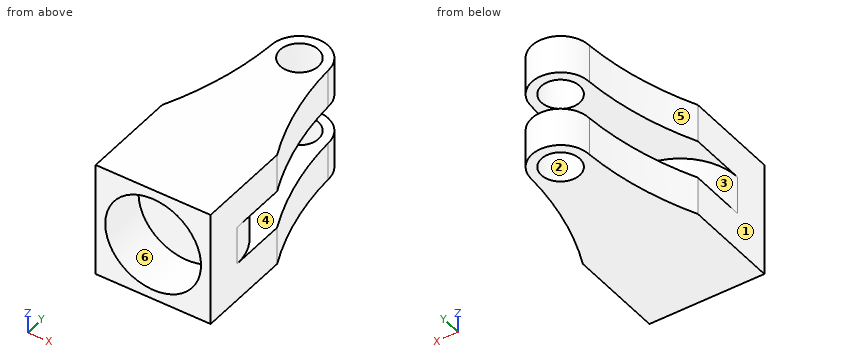
Autodesk Inventor part; units mm, degrees
ref_plane "Płaszczyzna konstrukcyjna2" through (-6, 5, 0) normal (0, 0, 1) x (1, 0, 0)
ref_plane "Płaszczyzna konstrukcyjna3" through (-6, -5, 0) normal (0, 0, 1) x (1, 0, 0)
ref_plane "YZ Plane" through (0, 0, 0) normal (1, 0, 0) x (0, 1, 0)
sketch "Szkic3" plane through (0, 0, 0) normal (0, 1, 0) x (-1, 0, 0)
  circle A0 centre (0, 0) radius 5
  line L0 (-6, -6) -> (6, -6)
  line L1 (6, -6) -> (6, 6)
  line L2 (6, 6) -> (-6, 6)
  line L3 (-6, 6) -> (-6, -6)
  line L4 (-6, -6) -> (6, 6) construction
  line L5 (6, -6) -> (-6, 6) construction
  dimension "d12" = 10
  dimension "d15" = 12
  dimension "d16" = 12
extrude "Wyciągnięcie proste3" add sketch "Szkic3" along normal mid plane 10
extrude "Wyciągnięcie proste4" add sketch "Szkic3" along normal blind 5 contours A0
ref_plane "Płaszczyzna konstrukcyjna2" through (-6, 5, 0) normal (0, 0, 1) x (1, 0, 0)
sketch "Szkic7" plane through (-6, 5, 0) normal (0, 0, 1) x (1, 0, 0)
  line L0 (0, -10) -> (0, 0)
  line L1 (0, 0) -> (12, 0)
  line L2 (12, 0) -> (6, 0)
  line L3 (6, 0) -> (6, 12) construction
  circle A0 centre (6, 12) radius 2
  line L4 (6, 12) -> (8, 12) construction
  line L5 (8, 12) -> (9, 12)
  line L6 (6, 12) -> (6, 14) construction
  line L7 (6, 14) -> (6, 15)
  arc A1 (9, 12) -> (6, 15) centre (6, 12) ccw
  arc A2 (9, 12) -> (12, 0) centre (41.9474, 13.8619) ccw
  line L8 (4, 12) -> (3, 12)
  arc A3 (6, 15) -> (3, 12) centre (6, 12) ccw
  arc A4 (0, 0) -> (3, 12) centre (-29.9474, 13.8619) ccw
  point P0 (6, -5)
  dimension "d61" = 12
  dimension "d62" = 4
  dimension "d63" = 1
  dimension "d64" = 2
  dimension "d65" = 1
  dimension "d66" = 3
  dimension "d67" = 33
  dimension "d68" = 1
  dimension "d69" = 2
  dimension "d70" = 3
  dimension "d71" = 33
extrude "Wyciągnięcie proste7" add sketch "Szkic7" along normal mid plane 12 contours A4 L8 A0 L5 A2 L1 | A3 L7 A0 L8 | A1 L5 A0 L7
ref_plane "Płaszczyzna konstrukcyjna3" through (-6, -5, 0) normal (0, 0, 1) x (1, 0, 0)
sketch "Szkic9" plane through (-6, -5, 0) normal (0, 0, 1) x (1, 0, 0)
  arc A0 (9, 22) -> (12, 10) centre (41.9474, 23.8619) ccw
  line L0 (0, 34) -> (12, 34)
  line L1 (12, 34) -> (12, 10)
  line L2 (12, 10) -> (0, 10)
  line L3 (0, 10) -> (0, 34)
  circle A1 centre (6, 22) radius 2
  line L4 (0, 34) -> (12, 10) construction
  line L5 (12, 34) -> (0, 10) construction
  point P0 (6, 5)
extrude "Wyciągnięcie proste9" cut sketch "Szkic9" along normal mid plane 4
fillet "Zaokrąglenie7" radius 6 2 edges at (6, 5, 0) (-6, 5, 0)
properties part number "Connector_hollow"
Verification items for the finished model (mm, model axes). Face numbers are marked on the shaded views. A direction names the side the tool comes from. Round coordinates to 2 decimals unless told otherwise and drop trailing zeros. Order: outer loops, then holes, each group sorted by start corner. A loop starts at its lowest first (then second) coordinate and runs counter-clockwise, first axis right, second up.
1) Cross-section at B-B, the plane y = -2.5. Record the cut outline in (x, z), plus the area to 3 significant figures.
Geometry says:
outline: (-6, -6) - (6, -6) - (6, 6) - (-6, 6) - close; hole circle Ø10 at (0, 0)
area: 65.5 mm2
2) Tool access check on the marked faces 4, 5 and 6. Record the directions out of +Z, -Z, +X, -X, +Y, -Y that give a thin tool (end or side, any length) a straight path to the whole face; none if there is none.
Geometry says:
face 4: +Y
face 5: +Z, -Z, -X, +Y
face 6: -Y
3) Draft check along Y on the marked faces 1, 2 and 3. Enter one of: +Y half, -Y half, draft (parallel to the pull), parting line (faces both ways), or undercut.
Geometry says:
face 1: draft
face 2: undercut
face 3: +Y half
4) Cross-section at A-A, the plane z = 4. Record the cut outline in (x, y), plus the area to 3 significant figures.
Geometry says:
outline: (-6, -5) - (-3, -5) - (-3, 0) - (3, 0) - (3, -5) - (6, -5) - (6, 5) arc R33 cw to (3, 17) arc R3 ccw to (-3, 17) arc R33 cw to (-6, 5) - close; hole circle Ø4 at (0, 17)
area: 190 mm2
5) Cross-section at C-C, the plane y = 18. Record the cut outline in (x, z), plus the area to 3 significant figures.
Geometry says:
outline: (-2.83, -6) - (-1.73, -6) - (-1.73, -2) - (-2.83, -2) - close; (-2.83, 2) - (-1.73, 2) - (-1.73, 6) - (-2.83, 6) - close; (1.73, -6) - (2.83, -6) - (2.83, -2) - (1.73, -2) - close; (1.73, 2) - (2.83, 2) - (2.83, 6) - (1.73, 6) - close
area: 17.5 mm2
6) Depth check by flat-ended pin: pin 1 (1 mm diameter, centred on y = 16.5, z = -1, fed in from -X); pin 2 (6 mm diameter, centred on x = 0, z = 0, fed in from -Y); pin 3 (2 mm diameter, centred on x = 2, z = 3, fed in from +Y). Enter the tip coordinate at first touch or a pass-through.
Geometry says:
pin 1: passes through
pin 2: stops at y = 0
pin 3: stops at y = 19.83
7) Cross-section at D-D, the plane x = -4. Record the cut outline in (y, z).
Geometry says:
outline: (-5, -6) - (10.59, -6) - (10.59, -2) - (3.47, -2) - (3.47, 2) - (10.59, 2) - (10.59, 6) - (-5, 6) - (-5, 3) - (0, 3) - (0, -3) - (-5, -3) - close
8) Material ranges on line 1 (Z direction, x = -0.25, y = 14.75); line 2 (X direction, y = 17, z = 5.2); line 3 (Y direction, x = 0, z = 4.35), recorded low to high.
Geometry says:
line 1: z = -6 to -2, 2 to 6
line 2: x = -3 to -2, 2 to 3
line 3: y = 0 to 15, 19 to 20
